from build123d import *

# Parameters (mm, degrees)
SKETCH1_R                 = 31.75
CENTERCIRCLEEXTRUDE_DEPTH = 19.558
SKETCH2_R                 = 80.01
BASEEXPAND_DEPTH          = 7.62
SKETCH3_R                 = 27.559
CENTERCUT_DEPTH           = 27.178
SKETCH4_R                 = 6.731
OUTERCIRCLECUT_DEPTH      = 7.62
SKETCH8_R                 = 80.01
STARFISHCUT_DEPTH         = 7.62
BATMAN_CUT_DEPTH          = 5.08
FILLET12_R                = 6.35


with BuildPart() as part:
    # Sketch1 → CenterCircleExtrude (new body)
    with BuildSketch(Plane(origin=(0, 0, 0), x_dir=(1, 0, 0), z_dir=(0, 1, 0))):
        with Locations(Location((0, 0, 0), (0, 0, 270))):
            Circle(SKETCH1_R)
    extrude(amount=CENTERCIRCLEEXTRUDE_DEPTH)

    # Sketch2 → BaseExpand (add)
    with BuildSketch(Plane.XZ):
        with Locations(Location((0, 0, 0), (0, 0, 90))):
            Circle(SKETCH2_R)
    extrude(amount=BASEEXPAND_DEPTH)

    # Sketch3 → CenterCut (cut)
    with BuildSketch(Plane(origin=(0, 19.558, 0), x_dir=(1, 0, 0), z_dir=(0, 1, 0))):
        with Locations(Location((0, 0, 0), (0, 0, 270))):
            Circle(SKETCH3_R)
    extrude(amount=-CENTERCUT_DEPTH, mode=Mode.SUBTRACT)

    # Sketch4 → OuterCircleCut (cut)
    with BuildSketch(Plane(origin=(0, 0, 0), x_dir=(1, 0, 0), z_dir=(0, 1, 0))):
        with Locations(Location((0, 55.118, 0), (0, 0, 270))):
            Circle(SKETCH4_R)
        with Locations(Location((52.420333065, 17.032398696, 0), (0, 0, 270))):
            Circle(SKETCH4_R)
        with Locations(Location((32.397547536, -44.591398696, 0), (0, 0, 270))):
            Circle(SKETCH4_R)
        with Locations(Location((-32.397547536, -44.591398696, 0), (0, 0, 270))):
            Circle(SKETCH4_R)
        with Locations(Location((-52.420333065, 17.032398696, 0), (0, 0, 270))):
            Circle(SKETCH4_R)
    extrude(amount=-OUTERCIRCLECUT_DEPTH, mode=Mode.SUBTRACT)

    # Sketch8 → StarfishCut (cut)
    with BuildSketch(Plane(origin=(0, 0, 0), x_dir=(1, 0, 0), z_dir=(0, 1, 0))):
        Circle(SKETCH8_R)
        with BuildLine():
            ThreePointArc((-60.451485692, 10.809361858), (-62.083067271, 20.172011359), (-55.259862746, 26.787534327))
            ThreePointArc((-55.259862746, 26.787534327), (-52.990125634, 27.176408575), (-50.691117004, 27.044162367))
            ThreePointArc((-50.691117004, 27.044162367), (-36.498445494, 28.482280038), (-22.436174146, 30.88074446))
            ThreePointArc((-22.436174146, 30.88074446), (-15.809618103, 43.513592992), (-10.056110229, 56.567222915))
            ThreePointArc((-10.056110229, 56.567222915), (-9.47145111, 58.794576379), (-8.400222382, 60.833055899))
            ThreePointArc((-8.400222382, 60.833055899), (0, 65.278), (8.400222382, 60.833055899))
            ThreePointArc((8.400222382, 60.833055899), (9.47145111, 58.794576379), (10.056110229, 56.567222915))
            ThreePointArc((10.056110229, 56.567222915), (15.809618103, 43.513592992), (22.436174146, 30.88074446))
            ThreePointArc((22.436174146, 30.88074446), (36.498445494, 28.482280038), (50.691117004, 27.044162367))
            ThreePointArc((50.691117004, 27.044162367), (52.990125634, 27.176408575), (55.259862746, 26.787534327))
            ThreePointArc((55.259862746, 26.787534327), (60.546685924, 23.130594267), (62.580333065, 17.032398696))
            ThreePointArc((62.580333065, 17.032398696), (62.033399971, 13.743851196), (60.451485692, 10.809361858))
            ThreePointArc((60.451485692, 10.809361858), (58.843804343, 9.160637981), (56.90613492, 7.916304043))
            ThreePointArc((56.90613492, 7.916304043), (46.26932683, -1.589400596), (36.302492346, -11.795394786))
            ThreePointArc((36.302492346, -11.795394786), (38.366897955, -25.910575851), (41.384943465, -39.853011375))
            ThreePointArc((41.384943465, -39.853011375), (42.22114982, -41.998632188), (42.552695773, -44.27744921))
            ThreePointArc((42.552695773, -44.27744921), (42.556334523, -44.434405209), (42.557547536, -44.591398696))
            ThreePointArc((42.557547536, -44.591398696), (38.241722309, -52.902308467), (28.960850446, -54.152502874))
            ThreePointArc((28.960850446, -54.152502874), (26.896020001, -53.132990748), (25.11381532, -51.674677951))
            ThreePointArc((25.11381532, -51.674677951), (12.786398515, -44.495896582), (0, -38.170699348))
            ThreePointArc((0, -38.170699348), (-12.786398515, -44.495896582), (-25.11381532, -51.674677951))
            ThreePointArc((-25.11381532, -51.674677951), (-26.896020001, -53.132990748), (-28.960850446, -54.152502874))
            ThreePointArc((-28.960850446, -54.152502874), (-38.369445699, -52.811011359), (-42.552695773, -44.27744921))
            ThreePointArc((-42.552695773, -44.27744921), (-42.22114982, -41.998632188), (-41.384943465, -39.853011375))
            ThreePointArc((-41.384943465, -39.853011375), (-38.366897955, -25.910575851), (-36.302492346, -11.795394786))
            ThreePointArc((-36.302492346, -11.795394786), (-46.26932683, -1.589400596), (-56.90613492, 7.916304043))
            ThreePointArc((-56.90613492, 7.916304043), (-58.843804343, 9.160637981), (-60.451485692, 10.809361858))
        make_face(mode=Mode.SUBTRACT)
    extrude(amount=-STARFISHCUT_DEPTH, mode=Mode.SUBTRACT)

    # Sketch14 → Batman Cut (cut)
    with BuildSketch(Plane(origin=(0, 0, 0), x_dir=(1, 0, 0), z_dir=(0, 1, 0))):
        with BuildLine():
            Line((-33.120038048, -5.061770157), (-29.510136252, -15.81140749))
            ThreePointArc((-29.510136252, -15.81140749), (-30.777930128, -18.361212827), (-33.327735465, -17.093418951))
            Line((-33.327735465, -17.093418951), (-36.937637261, -6.343781617))
            ThreePointArc((-36.937637261, -6.343781617), (-35.669843385, -3.793976281), (-33.120038048, -5.061770157))
        make_face()
        with BuildLine():
            Line((-15.048684103, 29.934855006), (-24.156675734, 23.17981376))
            ThreePointArc((-24.156675734, 23.17981376), (-26.973454567, 23.597624206), (-26.555644121, 26.414403039))
            Line((-26.555644121, 26.414403039), (-17.447652491, 33.169444285))
            ThreePointArc((-17.447652491, 33.169444285), (-14.630873657, 32.751633839), (-15.048684103, 29.934855006))
        make_face()
        with BuildLine():
            Line((23.819439787, 23.562527999), (14.580489593, 30.137320247))
            ThreePointArc((14.580489593, 30.137320247), (14.107418412, 32.94534664), (16.915444805, 33.418417821))
            Line((16.915444805, 33.418417821), (26.154394998, 26.843625573))
            ThreePointArc((26.154394998, 26.843625573), (26.62746618, 24.03559918), (23.819439787, 23.562527999))
        make_face()
        with BuildLine():
            Line((29.769907484, -15.372411842), (33.167913875, -4.553925517))
            ThreePointArc((33.167913875, -4.553925517), (35.692318639, -3.236280211), (37.009963945, -5.760684975))
            Line((37.009963945, -5.760684975), (33.611957554, -16.5791713))
            ThreePointArc((33.611957554, -16.5791713), (31.08755279, -17.896816606), (29.769907484, -15.372411842))
        make_face()
        with BuildLine():
            Line((-5.42062512, -33.063201006), (5.918408517, -32.951800999))
            ThreePointArc((5.918408517, -32.951800999), (7.951647645, -34.945477807), (5.957970836, -36.978716935))
            Line((5.957970836, -36.978716935), (-5.381062801, -37.090116942))
            ThreePointArc((-5.381062801, -37.090116942), (-7.414301928, -35.096440133), (-5.42062512, -33.063201006))
        make_face()
        with BuildLine():
            Line((-28.525313555, -22.027493495), (-12.265879706, -34.597736013))
            ThreePointArc((-12.265879706, -34.597736013), (-11.392472024, -41.423096527), (-18.217832537, -42.29650421))
            Line((-18.217832537, -42.29650421), (-34.477266386, -29.726261691))
            ThreePointArc((-34.477266386, -29.726261691), (-35.350674069, -22.900901178), (-28.525313555, -22.027493495))
        make_face()
        with BuildLine():
            Line((-29.764197885, 20.322315503), (-36.694767565, 0.974256428))
            ThreePointArc((-36.694767565, 0.974256428), (-42.91617334, -1.965556032), (-45.8559858, 4.255849744))
            Line((-45.8559858, 4.255849744), (-38.925416119, 23.603908818))
            ThreePointArc((-38.925416119, 23.603908818), (-32.704010344, 26.543721278), (-29.764197885, 20.322315503))
        make_face()
        with BuildLine():
            Line((10.130027615, 34.587375206), (-10.412733858, 35.1998596))
            ThreePointArc((-10.412733858, 35.1998596), (-15.131181768, 40.208316093), (-10.122725275, 44.926764002))
            Line((-10.122725275, 44.926764002), (10.420036198, 44.314279608))
            ThreePointArc((10.420036198, 44.314279608), (15.138484108, 39.305823116), (10.130027615, 34.587375206))
        make_face()
        with BuildLine():
            Line((36.024899257, 1.053857956), (30.259344125, 20.780453204))
            ThreePointArc((30.259344125, 20.780453204), (33.564588718, 26.815662007), (39.599797521, 23.510417414))
            Line((39.599797521, 23.510417414), (45.365352654, 3.783822167))
            ThreePointArc((45.365352654, 3.783822167), (42.060108061, -2.251386637), (36.024899257, 1.053857956))
        make_face()
        with BuildLine():
            Line((12.134584568, -33.93605517), (29.114037004, -22.356833218))
            ThreePointArc((29.114037004, -22.356833218), (35.875238414, -23.635325541), (34.596746091, -30.396526951))
            Line((34.596746091, -30.396526951), (17.617293654, -41.975748902))
            ThreePointArc((17.617293654, -41.975748902), (10.856092244, -40.697256579), (12.134584568, -33.93605517))
        make_face()
    extrude(amount=-BATMAN_CUT_DEPTH, mode=Mode.SUBTRACT)

    # Fillet12
    fillet12_edges = [part.edges().sort_by_distance(p)[0] for p in [
        (-22.436174146, -3.81, -30.88074446),
        (-36.302492346, -3.81, 11.795394786),
        (0, -3.81, 38.170699348),
        (36.302492346, -3.81, 11.795394786),
        (22.436174146, -3.81, -30.88074446),
    ]]
    fillet(fillet12_edges, radius=FILLET12_R)


solid = part.part
Model file for the job. Use its own axes, mm. A direction names the side the tool comes from. Give positions to 0.01 mm unless a question says otherwise; leave off trailing zeros. Order: outer loops, then holes, each group sorted by start corner. A loop starts at its lowest first (then second) coordinate and runs counter-clockwise, first axis right, second up. Notation, with made-up numbers: (46.25, 79.25) - (103.25, 79.25) arc R34 cw to (103.25, 114.25) - close; hole circle Ø9 at (46, 84.25). An arc over 180 degrees is marked (long way). One line per item, written item: value.
Item 1: Two-plate mould, pull along Z, no slides. Class faces 1 (the flat face through (26, 19.558, -10)), 2 (the cylindrical face through (-15.245, -3.757, -44.695)), 3 (the flat face through (-33.181, -2.504, -10.784)): released by +Z, released by -Z, zero draft, split by the parting line, or undercut.
Response values:
face 1: zero draft
face 2: released by -Z
face 3: undercut
Item 2: Wall check: line 1 (X direction, y = 6.25, z = 0.5); line 2 (X direction, y = -6, z = 47); line 3 (Z direction, x = -19, y = -3.5). Give the ranges that are in metal, low to high.
Response values:
line 1: -31.75 to -27.55, 27.55 to 31.75
line 2: -42.27 to -38.68, -26.11 to -17.31, 17.31 to 26.11, 38.68 to 42.27
line 3: -37.17 to -32.02, -27 to -19.96, 19.96 to 29.39, 41.69 to 47.97
Item 3: Slice it at A-A (z = -18.5). List the corners of the cut face in (x, y), then the cut area to 3 significant figures.
Response values:
outline: (-62.47, -7.62) - (-58.99, -7.62) - (-58.99, 0) - (-62.47, 0) - close; (-45.85, -7.62) - (-20.43, -7.62) - (-20.43, 19.56) - (-25.8, 19.56) - (-25.8, 0) - (-30.42, 0) - (-30.42, -5.08) - (-40.75, -5.08) - (-40.75, 0) - (-45.85, 0) - close; (20.43, -7.62) - (45.85, -7.62) - (45.85, 0) - (41.06, 0) - (41.06, -5.08) - (30.93, -5.08) - (30.93, 0) - (25.8, 0) - (25.8, 19.56) - (20.43, 19.56) - close; (58.99, -7.62) - (62.47, -7.62) - (62.47, 0) - (58.99, 0) - close
area: 547 mm2
Item 4: Pin check, flat tips, straight feed: pin 1 Ø4.5 at (x, z) = (34.5, -9) entering from +Y; pin 2 Ø4 at (y, z) = (-1, -53) entering from +X; pin 3 Ø10 at (x, y) = (-15.5, 6) entering from +Z. Stop position of each tip, or through.
Response values:
pin 1: y = 0
pin 2: x = 12.38
pin 3: z = 29.96
Item 5: Slice it at D-D (y = -2.75). Give the number of separate pieces and of enclosed holes in the cut face, then the cut area to 3 significant figures.
Response values:
separate pieces: 1
enclosed holes: 16
area: 3,450 mm2
Item 6: Slice it at C-C (z = -50). List the corners of the cut face in (x, y), then the cut area to 3 significant figures.
Response values:
outline: (-12.82, -7.62) - (-4.37, -7.62) - (-4.37, 0) - (-12.82, 0) - close; (4.37, -7.62) - (12.82, -7.62) - (12.82, 0) - (4.37, 0) - close
area: 129 mm2
Item 7: Tool access for faces 4 (the cylindrical face through (15.1, -3.8, -45)), 5 (the flat face through (-31.34, -2.5, 10.36)): list every direction of +Z, -Z, +X, -X, +Y, -Y with a clear straight run to the whole face (end or side of a thin tool).
Response values:
face 4: -Z, +X, +Y, -Y
face 5: +Y
Item 8: Slice it at B-B (y = 15.75). List the corners of the cut face in (x, z).
Response values:
outline: circle Ø63.5 at (0, 0); hole circle Ø55.12 at (0, 0)
